Work out the finished part from the listing and answer in its coordinate system (mm). A direction names the side the tool comes from. Give positions to 0.01 mm unless a question says otherwise; leave off trailing zeros. Loops run counter-clockwise (first coordinate to the right, second up) from the corner with the lowest first, then second, coordinate; pieces in that order, holes last. Notation, with made-up numbers: M 3,5 L 46,5 A28 ccw 46,43 Z; hole C 20,81 d7. An arc over 180 degrees is marked long. Write item = value, one per line. Start each with the question number.
1. Section A-A on x = 0 is taken. Determine the outline of the cut face in (y, z).
2. Section C-C on x = 15.5 is taken. Determine the outline of the cut face in (y, z), plus the area to 3 significant figures.
3. The mould has two halves that part along Y. Classify faces 1 (the face through (-14.39, -24.49, 3.45)), 2 (the face through (21, 0, 5)), 3 (the face through (0, 31, 5)), 4 (the face through (0, -31, 5)): released by +Y, released by -Y, zero draft, split by the parting line, or undercut.
4. Flat-ended cylindrical pins translate along their axes: pin 1 Ø6.5 at (x, y) = (-16, 6) entering from +Z; pin 2 Ø3.5 at (x, y) = (-15.5, -25.5) entering from +Z. Find the tip coordinate at first contact, or state that the pin passes through.
5. Section B-B on y = -10 is taken. Determine the outline of the cut face in (x, z), plus the area to 3 significant figures.
6. Consider L1, parallel to Y at x = 15.5, z = 8.8; L2, parallel to Y at x = 15.5, z = 5; L3, parallel to X at y = -26, z = 7.25. Determine where each line is inside the solid, lowest interval first. Write a range as [from, to].
7. For faces 5 (the face through (13.238, -27.234, 8.521)), 6 (the face through (17, 5.57, 3.45)), determine the directions among +Z, -Z, +X, -X, +Y, -Y from which every point of the face is accessible in a straight line to the end or side of a thin tool.
8. Section D-D on y = 5.5 is taken. Determine the outline of the cut face in (x, z).
```python
from build123d import *

# Parameters (mm, degrees)
SKETCH1_W           = 42
SKETCH1_H           = 62
BOSS_EXTRUDE1_DEPTH = 10
SKETCH2_R           = 1.5
SKETCH2_R_2         = 11
CUT_EXTRUDE1_DEPTH  = 11
SKETCH3_R           = 2.85
CUT_EXTRUDE2_DEPTH  = 3


with BuildPart() as part:
    # Sketch1 → Boss-Extrude1 (new body)
    with BuildSketch(Plane.XY):
        Rectangle(SKETCH1_W, SKETCH1_H)
    extrude(amount=BOSS_EXTRUDE1_DEPTH)

    # Sketch2 → Cut-Extrude1 (cut, through all)
    with BuildSketch(Plane(origin=(0, 0, 0), x_dir=(-1, 0, 0), z_dir=(0, 0, -1))):
        with Locations((15.5, 5.5)):
            Circle(SKETCH2_R)
        with Locations((15.5, -25.5)):
            Circle(SKETCH2_R)
        with Locations((-15.5, -25.5)):
            Circle(SKETCH2_R)
        with Locations((-15.5, 5.5)):
            Circle(SKETCH2_R)
        with Locations((0, -10)):
            Circle(SKETCH2_R_2)
    extrude(amount=-CUT_EXTRUDE1_DEPTH, mode=Mode.SUBTRACT)

    # Sketch3 → Cut-Extrude2 (cut)
    with BuildSketch(Plane.XY.offset(10)):
        with Locations((-15.5, 5.5)):
            Circle(SKETCH3_R)
        with Locations((15.5, 5.5)):
            Circle(SKETCH3_R)
        with Locations((15.5, -25.5)):
            Circle(SKETCH3_R)
        with Locations((-15.5, -25.5)):
            Circle(SKETCH3_R)
    extrude(amount=-CUT_EXTRUDE2_DEPTH, mode=Mode.SUBTRACT)


solid = part.part
```
Verdict:
q1.outline = M -31,0 L -21,0 L -21,10 L -31,10 Z; M 1,0 L 31,0 L 31,10 L 1,10 Z
q2.outline = M -31,0 L -27,0 L -27,7 L -28.35,7 L -28.35,10 L -31,10 Z; M -24,0 L 4,0 L 4,7 L 2.65,7 L 2.65,10 L -22.65,10 L -22.65,7 L -24,7 Z; M 7,0 L 31,0 L 31,10 L 8.35,10 L 8.35,7 L 7,7 Z
q2.area = 544 mm2
q3.face_1 = undercut
q3.face_2 = zero draft
q3.face_3 = released by +Y
q3.face_4 = released by -Y
q4.pin_1 = 10
q4.pin_2 = 7
q5.outline = M -21,0 L -11,0 L -11,10 L -21,10 Z; M 11,0 L 21,0 L 21,10 L 11,10 Z
q5.area = 200 mm2
q6.L1 = [-31, -28.35], [-22.65, 2.65], [8.35, 31]
q6.L2 = [-31, -27], [-24, 4], [7, 31]
q6.L3 = [-21, -18.31], [-12.69, 12.69], [18.31, 21]
q7.face_5 = +Z
q7.face_6 = +Z, -Z
q8.outline = M -21,0 L -17,0 L -17,7 L -18.35,7 L -18.35,10 L -21,10 Z; M -14,0 L 14,0 L 14,7 L 12.65,7 L 12.65,10 L -12.65,10 L -12.65,7 L -14,7 Z; M 17,0 L 21,0 L 21,10 L 18.35,10 L 18.35,7 L 17,7 Z
